Geometry check sheet. Reference: the model listing, model coordinates, mm. A direction names the side the tool comes from. Coordinates: 2 decimals unless noted, no trailing zeros. Write each loop counter-clockwise with the first axis right and the second up, starting at its lowest first coordinate (ties: lowest second). Pieces come first, ordered by that corner, then holes. Notation, with made-up numbers: M 54.25,35 L 75.25,35 A20 cw 75.25,63 Z; hole C -4.5,-30 d8. An arc over 180 degrees is marked long. Write each question's results on one line, items separated by ' | '.
```python
from build123d import *

# Parameters (mm, degrees)
SKETCH_W        = 16
SKETCH_H        = 39
PAD_DEPTH       = 13
POCKET_DEPTH    = 39.001
POCKET001_DEPTH = 16.001


with BuildPart() as part:
    # Sketch → Pad (new body)
    with BuildSketch(Plane.XY):
        Rectangle(SKETCH_W, SKETCH_H)
    extrude(amount=PAD_DEPTH)

    # Sketch001 (on Face1 of Pad) → Pocket (cut, through all)
    with BuildSketch(Plane(origin=(0, 19.5, 0), x_dir=(-1, 0, 0), z_dir=(0, 1, 0))):
        Polygon((-5, 5.5), (5, 5.5), (5, 2), (2.5, 2), (2.5, 0), (-2.5, 0), (-2.5, 2), (-5, 2), align=None)
    extrude(amount=-POCKET_DEPTH, mode=Mode.SUBTRACT)

    # Sketch002 (on Face11 of Pocket) → Pocket001 (cut, through all)
    with BuildSketch(Plane.YZ.offset(8)):
        Polygon((-13.5, 13), (-13.5, 11), (-16.5, 11), (-16.5, 7), (16.5, 7), (16.5, 11), (13.5, 11), (13.5, 13), align=None)
    extrude(amount=-POCKET001_DEPTH, mode=Mode.SUBTRACT)


solid = part.part
```
Q1. Sectioned sample at C-C on z = 3. Record the cut outline in (x, y).
Geometry check:
outline: M -8,-19.5 L -5,-19.5 L -5,19.5 L -8,19.5 Z; M 5,-19.5 L 8,-19.5 L 8,19.5 L 5,19.5 Z
Q2. Sectioned sample at B-B on y = -14.5. Record the cut outline in (x, z).
Geometry check:
outline: M -8,0 L -2.5,0 L -2.5,2 L -5,2 L -5,5.5 L 5,5.5 L 5,2 L 2.5,2 L 2.5,0 L 8,0 L 8,7 L -8,7 Z; M -8,11 L 8,11 L 8,13 L -8,13 Z
Q3. Sectioned sample at D-D on x = -6.5. Record the cut outline in (y, z), and give its area (3 significant figures).
Geometry check:
outline: M -19.5,0 L 19.5,0 L 19.5,13 L 13.5,13 L 13.5,11 L 16.5,11 L 16.5,7 L -16.5,7 L -16.5,11 L -13.5,11 L -13.5,13 L -19.5,13 Z | area: 321 mm2
Q4. Mould release check, pull along Z, two halves, no side actions. Record for faces 1 (the flat face through (2.5, 0, 1)), 2 (the flat face through (5, 0, 4)), 3 (the flat face through (-5, 0, 0)), 4 (the flat face through (0, -16, 13)): pulls with the +Z half, pulls with the -Z half, needs draft (parallel to the pull), parting line crosses it, or undercut.
Geometry check:
face 1: needs draft | face 2: undercut | face 3: pulls with the -Z half | face 4: pulls with the +Z half
Q5. Sectioned sample at A-A on x = -4.5. Record the cut outline in (y, z).
Geometry check:
outline: M -19.5,0 L 19.5,0 L 19.5,2 L -19.5,2 Z; M -19.5,5.5 L 19.5,5.5 L 19.5,13 L 13.5,13 L 13.5,11 L 16.5,11 L 16.5,7 L -16.5,7 L -16.5,11 L -13.5,11 L -13.5,13 L -19.5,13 Z
Q6. Scan lines: probe 1 along Z at (x, y) = (4.75, -14); probe 2 along Z at (x, y) = (6.5, -15); probe 3 along Z at (x, y) = (3.5, 0). Record each from-to range of solid material in increasing order.
Geometry check:
probe 1: z = 0 to 2, 5.5 to 7, 11 to 13 | probe 2: z = 0 to 7, 11 to 13 | probe 3: z = 0 to 2, 5.5 to 7
Q7. Access from +Z, -Z, +X, -X, +Y, -Y to the whole of each face (thin tool, end or side, straight path). Record for faces 5 (the flat face through (0, -13.5, 12)), 6 (the flat face through (-2.5, 0, 1)), 7 (the flat face through (0, 0, 5.5)), 8 (the flat face through (0, 15, 11)).
Geometry check:
face 5: +Z, +X, -X | face 6: -Z, +Y, -Y | face 7: +Y, -Y | face 8: +X, -X
Q8. Depth check by flat-ended pin: P1, Ø1.5, axis at x = -1.5, y = 15, coming from the -Z side; P2, Ø3, axis at x = -3.5, y = 9.5, coming from the +Z side. Enter the tip coordinate at first touch or a pass-through.
Geometry check:
P1: stops at z = 5.5 | P2: stops at z = 7
